CAD build for the part. Positions are in the model's coordinates, mm. A direction names the side the tool comes from. Coordinates: 2 decimals unless noted, no trailing zeros. Loops run counter-clockwise (first coordinate to the right, second up) from the corner with the lowest first, then second, coordinate; pieces in that order, holes last. Notation, with made-up numbers: (-24.5, 56.5) -> (-9.5, 56.5) arc R20 cw to (-9.5, 85.5) -> close; hole circle Ø4 at (-38, 61.25). An arc over 180 degrees is marked (long way). Answer as a JSON object with one key per item and string values. Group by question number.
from build123d import *

# Parameters (mm, degrees)
BOSS_EXTRU_1_DEPTH      = 60
ENL_V_MAT_EXTRU_1_DEPTH = 60
CONG_1_R                = 10
ENL_V_MAT_EXTRU_2_DEPTH = 60
CONG_2_R                = 10
ESQUISSE4_W             = 15
ESQUISSE4_H             = 60
BOSS_EXTRU_2_DEPTH      = 5
BOSS_EXTRU_3_START      = -32.5
ESQUISSE5_R             = 7.789836859
ESQUISSE5_R_2           = 5.25
BOSS_EXTRU_3_DEPTH      = 5
ESQUISSE6_W             = 10
ESQUISSE6_H             = 5
BOSS_EXTRU_4_DEPTH      = 5
CONG_3_R                = 11


with BuildPart() as part:
    # Esquisse1 → Boss.-Extru.1 (new body)
    with BuildSketch(Plane.XY):
        Polygon((0, 0), (29.226497308, 50.621778265), (100.773502692, 50.621778265), (130, 0), (140, 0), (105, 60.621778265), (25, 60.621778265), (-10, 0), align=None)
    extrude(amount=BOSS_EXTRU_1_DEPTH)

    # Esquisse2 → Enlèv. mat.-Extru.1 (cut)
    with BuildSketch(Plane(origin=(0, 0, 0), x_dir=(-1, 0, 0), z_dir=(0, 0, -1))):
        with BuildLine():
            Line((-105, 60.621778265), (-25, 60.621778265))
            ThreePointArc((-25, 60.621778265), (-65, 55.979286299), (-105, 60.621778265))
        make_face()
    extrude(amount=-ENL_V_MAT_EXTRU_1_DEPTH, mode=Mode.SUBTRACT)

    # Congé1
    cong_1_edges = [part.edges().sort_by_distance(p)[0] for p in [
        (25, 60.621778265, 30),
        (105, 60.621778265, 30),
    ]]
    fillet(cong_1_edges, radius=CONG_1_R)

    # Esquisse3 → Enlèv. mat.-Extru.2 (cut)
    with BuildSketch(Plane(origin=(0, 0, 0), x_dir=(1, 0, 0), z_dir=(0, 1, 0))):
        with BuildLine():
            Line((70, -15), (70, -45))
            ThreePointArc((70, -45), (65, -50), (60, -45))
            Line((60, -45), (60, -15))
            ThreePointArc((60, -15), (65, -10), (70, -15))
        make_face()
    extrude(amount=ENL_V_MAT_EXTRU_2_DEPTH, mode=Mode.SUBTRACT)

    # Congé2
    cong_2_edges = [part.edges().sort_by_distance(p)[0] for p in [
        (100.773502692, 50.621778265, 30),
        (29.226497308, 50.621778265, 30),
    ]]
    fillet(cong_2_edges, radius=CONG_2_R)

    # Esquisse4 → Boss.-Extru.2 (add)
    with BuildSketch(Plane.XZ):
        with Locations((-7.5, 30)):
            Rectangle(ESQUISSE4_W, ESQUISSE4_H)
        with Locations((137.5, 30)):
            Rectangle(ESQUISSE4_W, ESQUISSE4_H)
    extrude(amount=-BOSS_EXTRU_2_DEPTH)

    # Esquisse5 → Boss.-Extru.3 (add)
    # profile 1 of 3: a face of its own
    with BuildSketch(Plane.XY.offset(60).offset(BOSS_EXTRU_3_START)):
        with BuildLine():
            Line((115.375109784, 42.651560984), (141.355871898, 57.651560984))
            ThreePointArc((141.355871898, 57.651560984), (161.846252955, 52.161179927), (156.355871898, 31.670798871))
            Line((156.355871898, 31.670798871), (130.375109784, 16.670798871))
            Line((130.375109784, 16.670798871), (115.375109784, 42.651560984))
        make_face()
        with Locations(Location((148.855871898, 44.661179927, 0), (0, 0, 180))):
            Circle(ESQUISSE5_R, mode=Mode.SUBTRACT)
    # profile 2 of 3: a face of its own
    with BuildSketch(Plane.XY.offset(60).offset(BOSS_EXTRU_3_START)):
        with BuildLine():
            Line((14.624890216, 42.651560984), (-0.375109784, 16.670798871))
            Line((-0.375109784, 16.670798871), (-26.355871898, 31.670798871))
            ThreePointArc((-26.355871898, 31.670798871), (-31.846252955, 52.161179927), (-11.355871898, 57.651560984))
            Line((-11.355871898, 57.651560984), (14.624890216, 42.651560984))
        make_face()
        with Locations((-18.855871898, 44.661179927)):
            Circle(ESQUISSE5_R, mode=Mode.SUBTRACT)
    # profile 3 of 3: a face of its own
    with BuildSketch(Plane.XY.offset(60).offset(BOSS_EXTRU_3_START)):
        with BuildLine():
            Line((45, 72.128262536), (45, 57.128262536))
            ThreePointArc((45, 57.128262536), (65, 55.979286299), (85, 57.128262536))
            Line((85, 57.128262536), (85, 72.128262536))
            ThreePointArc((85, 72.128262536), (65, 92.128262536), (45, 72.128262536))
        make_face()
        with Locations((65, 72.128262536)):
            Circle(ESQUISSE5_R_2, mode=Mode.SUBTRACT)
    extrude(amount=BOSS_EXTRU_3_DEPTH)

    # Esquisse6 → Boss.-Extru.4 (add)
    with BuildSketch(Plane.XZ.offset(-50.621778265)):
        with Locations((65, 30)):
            Rectangle(ESQUISSE6_W, ESQUISSE6_H)
    extrude(amount=-BOSS_EXTRU_4_DEPTH)

    # Congé3
    # the kernel refuses this fillet: 11 mm, written as the material it adds along each edge
    with BuildSketch(Plane(origin=(85, 57.128262536, 27.5), x_dir=(0.9883685049856061, 0.15207793512708467, 0), z_dir=(0, 0, 1))) as cong_3_piece_1:
        with BuildLine():
            CenterArc((12.820682636, 10.992120116), CONG_3_R, 171.25263481, 100.916203285)
            Line((1.948629081, 12.664977402), (0.861423726, 12.832263131))
            ThreePointArc((0.861423726, 12.832263131), (-0.112841396, 6.499766826), (-1.087205355, 0.167285729))
            Line((-1.087205355, 0.167285729), (-0.041678758, -1.099210117))
            ThreePointArc((-0.041678758, -1.099210117), (13.278085549, -1.099131399), (13.278598986, -1.099212012))
            Line((13.278598986, -1.099212012), (13.236970227, 0))
        make_face()
    extrude(amount=5)
    with BuildSketch(Plane(origin=(45, 57.128262536, 27.5), x_dir=(-0.9883685049856065, 0.1520779351270834, 0), z_dir=(0, 0, 1))) as cong_3_piece_2:
        with BuildLine():
            CenterArc((12.820682636, -10.992120116), CONG_3_R, 87.831161905, 100.916203285)
            Line((1.948629081, -12.664977402), (0.861423726, -12.832263131))
            ThreePointArc((0.861423726, -12.832263131), (-0.112841396, -6.499766826), (-1.087205355, -0.167285729))
            Line((-1.087205355, -0.167285729), (-0.041678758, 1.099210117))
            ThreePointArc((-0.041678758, 1.099210117), (13.278085549, 1.099131399), (13.278598986, 1.099212012))
            Line((13.278598986, 1.099212012), (13.236970227, 0))
        make_face()
    extrude(amount=5)


solid = part.part
Item 1: Band-saw the part on A-A, the plane x = 65. List the corners of the cut face in (y, z).
Item 2: 3-axis set-ups, long thin cutter, end or side, ignore diameter. For faces 1 (the flat face through (62.7, 77.3, 27.5)), 2 (the flat face through (65, 66, 32.5)), 3 (the flat face through (116.646, 23.13, 29.58)), 4 (the flat face through (-9, 38, 27.5)): which of +Z, -Z, +X, -X, +Y, -Y reach the whole face in a straight line?
Item 3: Band-saw the part on C-C, the plane z = 52.5. List the corners of the cut face in (x, y).
Item 4: Band-saw the part on D-D, the plane y = 65. List the corners of the cut face in (x, z), and give its area (3 significant figures).
Item 5: Drill centre lines: L1, parallel to Y at x = 36, z = 28; L2, parallel to Z at x = 45, y = 67.5; L3, parallel to X at y = 30.5, z = 33. Where is each one in solid material? Low to high.
Item 6: Flat gauge pins, fed straight in: P1, Ø18, axis at x = 76.5, y = 83, coming from the +Z side; P2, Ø1.8, axis at y = 70.5, z = 31, coming from the -X side; P3, Ø1, axis at y = 56, z = 34.5, coming from the -X side. Where does each tip first touch, or does it go through?
Item 7: Pull direction X, two halves, no side cores. Call faces 5 (the flat face through (-11, 5, 30)), 6 (the cylindrical face through (65.44, 92.123, 29.965)), 7 (the flat face through (1.45, 50.26, 29.96)): +X half, -X half, draft (parallel to the pull), parting line (faces both ways), or undercut.
Item 8: Band-saw the part on B-B, the plane z = 34.5. List the corners of the cut face in (x, y), and give its area (3 significant figures).
Reply:
{
 "1": {"outline": "(50.62, 0) -> (55.98, 0) -> (55.98, 10) -> (50.62, 10) -> close; (50.62, 27.5) -> (55.62, 27.5) -> (55.62, 32.5) -> (50.62, 32.5) -> close; (50.62, 50) -> (55.98, 50) -> (55.98, 60) -> (50.62, 60) -> close; (55.98, 27.5) -> (66.88, 27.5) -> (66.88, 32.5) -> (55.98, 32.5) -> close; (77.38, 27.5) -> (92.13, 27.5) -> (92.13, 32.5) -> (77.38, 32.5) -> close"},
 "2": {"face 1": "-Z, +Y", "face 2": "+Z, +Y", "face 3": "+Z, -Z, -Y", "face 4": "-Z, -X, +Y"},
 "3": {"outline": "(-15, 0) -> (0, 0) -> (26.34, 45.62) arc R10 cw to (35, 50.62) -> (95, 50.62) arc R10 cw to (103.66, 45.62) -> (130, 0) -> (145, 0) -> (145, 5) -> (137.11, 5) -> (108.64, 54.32) arc R10 ccw to (98.08, 59.14) arc R174.64 cw to (31.92, 59.14) arc R10 ccw to (21.36, 54.32) -> (-7.11, 5) -> (-15, 5) -> close"},
 "4": {"outline": "(43.83, 27.5) -> (86.17, 27.5) -> (86.17, 32.5) -> (43.83, 32.5) -> close", "area": "212 mm²"},
 "5": {"L1": "50.62 to 59.13", "L2": "27.5 to 32.5", "L3": "7.61 to 17.61, 112.39 to 122.39"},
 "6": {"P1": "z = 32.5", "P2": "x = 44.99", "P3": "x = 22.16"},
 "7": {"face 5": "draft", "face 6": "parting line", "face 7": "undercut"},
 "8": {"outline": "(-15, 0) -> (0, 0) -> (26.34, 45.62) arc R10 cw to (35, 50.62) -> (60, 50.62) -> (60, 56.05) arc R174.64 cw to (31.92, 59.14) arc R10 ccw to (21.36, 54.32) -> (-7.11, 5) -> (-15, 5) -> close; (70, 50.62) -> (95, 50.62) arc R10 cw to (103.66, 45.62) -> (130, 0) -> (145, 0) -> (145, 5) -> (137.11, 5) -> (108.64, 54.32) arc R10 ccw to (98.08, 59.14) arc R174.64 cw to (70, 56.05) -> close", "area": "1,620 mm²"}
}
